```python
from build123d import *

# Parameters (mm, degrees)
F1_DEPTH    = 25
F2_R        = 3
F3_T1_DEPTH = 150
F3_T4_ANGLE = 90


# Not quite as in the source:
# - a fillet or chamfer that OpenCascade refuses, or shapes differently, is made with other operations: its cross-section is extruded or revolved along the edge and cut away or added


with BuildPart() as f1:
    # F0 (on Right) → F1 (new body)
    with BuildSketch(Plane.YZ):
        Polygon((0, 2000), (0, 0), (1200, 0), (1200, 800), (900, 800), (900, 2000), align=None)
    extrude(amount=F1_DEPTH)

    # F2
    f2_edges = [f1.edges().sort_by_distance(p)[0] for p in [
        (25, 0, 1000),
        (25, 600, 0),
        (25, 1200, 400),
        (25, 1050, 800),
        (25, 900, 1400),
        (25, 450, 2000),
    ]]
    fillet(f2_edges, radius=F2_R)

    # F3: fillet of radius 50 on 1 edges, made by hand

    # F3_s2 → F3_t1 (cut)
    with BuildSketch(Plane.YZ.offset(-125)):
        with BuildLine():
            ThreePointArc((850, 2000), (885.3553390593, 1985.3553390593), (900, 1950))
            Line((900, 1950), (900, 2000))
            Line((900, 2000), (850, 2000))
        make_face()
    extrude(amount=F3_T1_DEPTH, mode=Mode.SUBTRACT)

    # F3_s3 → F3_t4 (revolve, cut)
    with BuildSketch(Plane.XY.offset(1950)):
        with BuildLine():
            ThreePointArc((25, 897), (24.1213203436, 899.1213203436), (22, 900))
            Line((22, 900), (25, 900))
            Line((25, 900), (25, 897))
        make_face()
    revolve(axis=Axis((25, 850, 1950), (1, 0, 0)), revolution_arc=F3_T4_ANGLE, mode=Mode.SUBTRACT)


solid = f1.part
```
For this review, take the finished solid that the model builds, in its own axes (mm). Coordinates: 2 decimals unless noted, no trailing zeros. Loops run counter-clockwise (first coordinate to the right, second up) from the corner with the lowest first, then second, coordinate; pieces in that order, holes last.
1. Add section B-B, the plane y = 1015. Give the boundary of the cut face in (x, z).
2. Insertion check: P1, Ø11, axis at x = 16, z = 1322, coming from the +Y side; P2, Ø4, axis at x = 6, y = 990.5, coming from the +Z side. Each pin has a flat end and moves straight along its axis. Give the tip position at first contact, or say it passes through.
3. For line 1 (Y direction, x = 1.25, z = 1666); line 2 (Z direction, x = 4.25, y = 1149.5); line 3 (Y direction, x = 22.75, z = 1315), list the stretches that pass through material, from the lowest coordinate up.
4. Add section C-C, the plane z = 1836.5. Give the boundary of the cut face in (x, y), then the cut area to 3 significant figures.
5. Add section A-A, the plane x = 17. Give the boundary of the cut face in (y, z).
Result:
1. outline: (0, 0) - (22, 0) arc R3 ccw to (25, 3) - (25, 797) arc R3 ccw to (22, 800) - (0, 800) - close
2. P1: stops at y = 900
2. P2: stops at z = 800
3. line 1: y = 0 to 900
3. line 2: z = 0 to 800
3. line 3: y = 0.1 to 899.9
4. outline: (0, 0) - (22, 0) arc R3 ccw to (25, 3) - (25, 897) arc R3 ccw to (22, 900) - (0, 900) - close
4. area: 22,500 mm2
5. outline: (0, 0) - (1200, 0) - (1200, 800) - (900, 800) - (900, 1950) arc R50 ccw to (850, 2000) - (0, 2000) - close
